Verification items for this drawing (mm, ordinates from the low corner). A direction names the side the tool comes from. Give positions to 0.01 mm unless a question says otherwise; leave off trailing zeros. Order: outer loops, then holes, each group sorted by start corner. A loop starts at its lowest first (then second) coordinate and runs counter-clockwise, first axis right, second up. Notation, with made-up numbers: M 65.25,89.25 L 83.25,89.25 A30 cw 83.25,118.25 Z; hole C -20.75,28 d11. An arc over 180 degrees is marked long. Return JSON: item names as keys, results as strings. Group by question number.
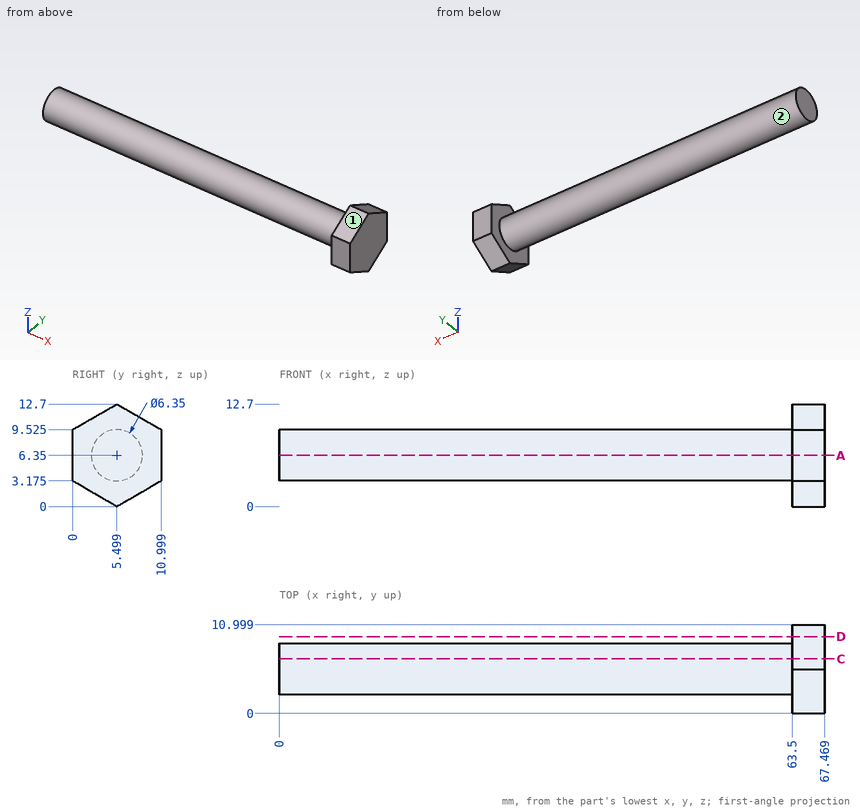
1) Sectioned sample at D-D on y = 9.5. Record the boundary of the cut face in (x, z), then the cut area to 3 significant figures.
2) Material ranges on line 1 along X through (y, z) = (1.25, 9.75); line 2 along Z through (x, y) = (11, 6.5); line 3 along Y through (x, z) = (53.5, 5) (1 decimal), recorded low to high.
3) Sectioned sample at C-C on y = 6.75. Record the boundary of the cut face in (x, z), then the cut area to 3 significant figures.
4) Tool access check on the marked faces 1 and 2. Record the directions out of +Z, -Z, +X, -X, +Y, -Y that give a thin tool (end or side, any length) a straight path to the whole face; none if there is none.
5) Depth check by flat-ended pin: P1, Ø1.5, axis at x = 42.5, z = 4, coming from the +Y side; P2, Ø3, axis at x = 32, y = 2, coming from the +Z side; P3, Ø1, axis at x = 50.5, z = 5, coming from the -Y side. Enter the tip coordinate at first touch or a pass-through.
6) Sectioned sample at A-A on z = 6.35. Record the boundary of the cut face in (x, y) (1 decimal).
Reply:
{
 "1": {"outline": "M 63.5,2.31 L 67.47,2.31 L 67.47,10.39 L 63.5,10.39 Z", "area": "32.1 mm^2"},
 "2": {"line 1": "63.5 to 67.47", "line 2": "3.34 to 9.36", "line 3": "2.6 to 8.4"},
 "3": {"outline": "M 0,3.43 L 63.5,3.43 L 63.5,0.72 L 67.47,0.72 L 67.47,11.98 L 63.5,11.98 L 63.5,9.27 L 0,9.27 Z", "area": "415 mm^2"},
 "4": {"face 1": "+Z, +X, -X, -Y", "face 2": "-X"},
 "5": {"P1": "y = 8.24", "P2": "z = 8.82", "P3": "y = 2.44"},
 "6": {"outline": "M 0,2.3 L 63.5,2.3 L 63.5,0 L 67.5,0 L 67.5,11 L 63.5,11 L 63.5,8.7 L 0,8.7 Z"}
}
